Could you check a few things on this drawing? It's one solid part, dimensions in mm from its lowest x, y, z. Give positions to 0.01 mm unless a question says otherwise; leave off trailing zeros. Loops run counter-clockwise (first coordinate to the right, second up) from the corner with the lowest first, then second, coordinate; pieces in that order, holes last. Notation, with made-up numbers: (-23.5, -39.5) -> (16.5, -39.5) arc R30 ccw to (16.5, -13.5) -> close; hole circle Ø2 at (49.25, 77.5). An arc over 180 degrees is marked (long way). One line per question, with ' | ' between items.
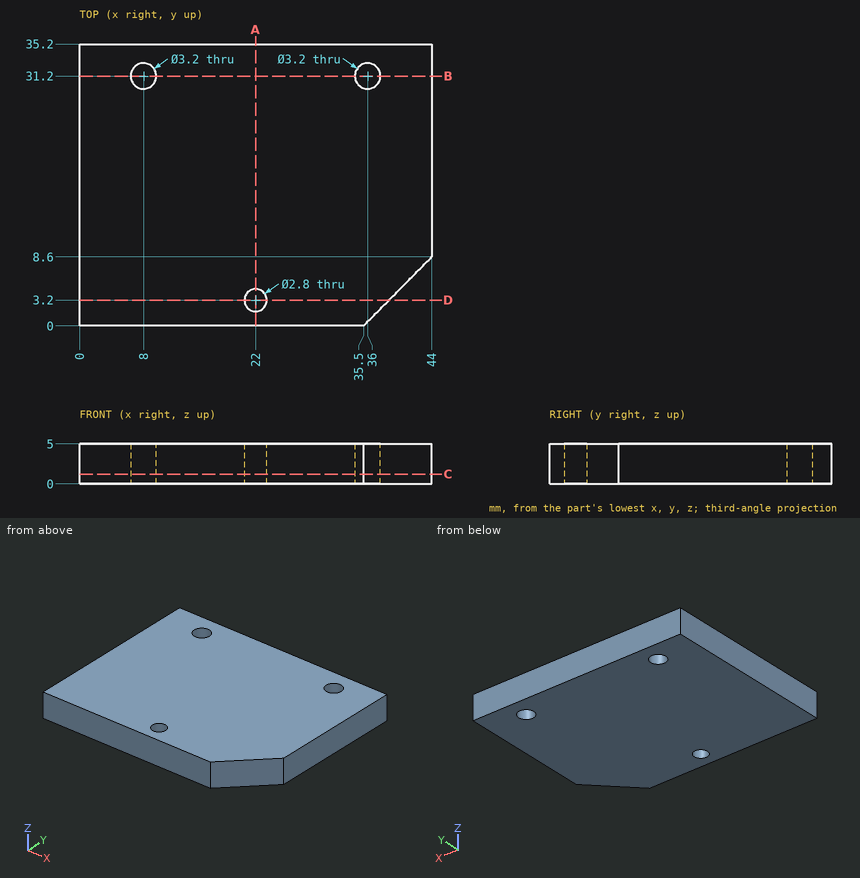
Q1. If we section it at D-D (y = 3.2): Write out the boundary of the cut face in (x, z).
Entries:
outline: (0, 0) -> (20.6, 0) -> (20.6, 5) -> (0, 5) -> close; (23.4, 0) -> (38.66, 0) -> (38.66, 5) -> (23.4, 5) -> close
Q2. If I drill on probe 1 along Y at (x, z) = (8, 1.3); probe 2 along Y at (x, z) = (22, 0.65); probe 3 along X at (y, z) = (32.5, 3.25), over which ranges is the centre line in solid material (lowest first)? Write a range as from..to.
Entries:
probe 1: 0..29.6, 32.8..35.2 | probe 2: 0..1.8, 4.6..35.2 | probe 3: 0..7.07, 8.93..35.07, 36.93..44
Q3. If we section it at A-A (x = 22): Write out the boundary of the cut face in (y, z), plus the area to 3 significant figures.
Entries:
outline: (0, 0) -> (1.8, 0) -> (1.8, 5) -> (0, 5) -> close; (4.6, 0) -> (35.2, 0) -> (35.2, 5) -> (4.6, 5) -> close | area: 162 mm²
Q4. If we section it at C-C (z = 1.2): Write out the boundary of the cut face in (x, y).
Entries:
outline: (0, 0) -> (35.5, 0) -> (44, 8.6) -> (44, 35.2) -> (0, 35.2) -> close; hole circle Ø3.2 at (8, 31.2); hole circle Ø2.8 at (22, 3.2); hole circle Ø3.2 at (36, 31.2)
Q5. If we section it at B-B (y = 31.2): Write out the boundary of the cut face in (x, z).
Entries:
outline: (0, 0) -> (6.4, 0) -> (6.4, 5) -> (0, 5) -> close; (9.6, 0) -> (34.4, 0) -> (34.4, 5) -> (9.6, 5) -> close; (37.6, 0) -> (44, 0) -> (44, 5) -> (37.6, 5) -> close
